Read the model definition and answer for the solid it produces. Units are mm, in the model's axes. A direction names the side the tool comes from. Round coordinates to 2 decimals unless told otherwise and drop trailing zeros. Write each loop counter-clockwise with the first axis right and the second up, starting at its lowest first coordinate (ties: lowest second). Pieces come first, ordered by that corner, then holes.
from build123d import *

# Parameters (mm, degrees)
F0_W     = 10
F0_H     = 10
F0_R     = 2.526739
F1_DEPTH = 1
F2_W     = 10
F2_H     = 1
F3_DEPTH = 9
F4_W     = 10
F4_H     = 1
F5_DEPTH = 9


with BuildPart() as f1:
    # F0 (on Top) → F1 (new body)
    with BuildSketch(Plane.XY):
        Rectangle(F0_W, F0_H)
        Circle(F0_R, mode=Mode.SUBTRACT)
    extrude(amount=F1_DEPTH)

    # F2 (on face) → F3 (join)
    with BuildSketch(Plane.XY.offset(1)):
        with Locations((0, 4.5)):
            Rectangle(F2_W, F2_H)
    extrude(amount=F3_DEPTH)

    # F4 (on face) → F5 (join)
    with BuildSketch(Plane.XZ.offset(-4)):
        with Locations((0, 9.5)):
            Rectangle(F4_W, F4_H)
    extrude(amount=F5_DEPTH)


solid = f1.part
Q1. Section D-D (x = -4) is taken. Determine the outline of the cut face in (y, z).
Verdict:
outline: (-5, 0) - (5, 0) - (5, 10) - (-5, 10) - (-5, 9) - (4, 9) - (4, 1) - (-5, 1) - close
Q2. Section B-B (x = 0) is taken. Determine the outline of the cut face in (y, z).
Verdict:
outline: (-5, 0) - (-2.53, 0) - (-2.53, 1) - (-5, 1) - close; (-5, 9) - (4, 9) - (4, 1) - (2.53, 1) - (2.53, 0) - (5, 0) - (5, 10) - (-5, 10) - close
Q3. A flat-ended cylindrical pin translates along its axis: pin 1 Ø4 at (x, z) = (-2, 4.5) entering from -Y. Find the tip coordinate at first contact, or state that the pin passes through.
Verdict:
pin 1: stops at y = 4
Q4. Section C-C (y = 2.75) is taken. Determine the outline of the cut face in (x, z).
Verdict:
outline: (-5, 0) - (5, 0) - (5, 1) - (-5, 1) - close; (-5, 9) - (5, 9) - (5, 10) - (-5, 10) - close
Q5. Which of the six approach directions +Z, -Z, +X, -X, +Y, -Y give full straight-line access (tool end or side, diameter ignored) to faces 5 (the flat face through (-0.1, -5, 0.5)), 6 (the flat face through (0, 0, 9))?
Verdict:
face 5: +Z, -Z, +X, -X, -Y
face 6: +X, -X, -Y
Q6. Straight lines are drawn through the part: probe 1 along Z at (x, y) = (4.25, 1.5); probe 2 along Y at (x, z) = (-2.75, 7.5); probe 3 along X at (y, z) = (2, 0.5). For each, find the intervals that lie inside material, in ascending order.
Verdict:
probe 1: z = 0 to 1, 9 to 10
probe 2: y = 4 to 5
probe 3: x = -5 to -1.54, 1.54 to 5
Q7. Determine the mould class of faces 1 (the flat face through (5, 4.5, 5.3)), 2 (the flat face through (-5, 4.5, 5.3)), 3 (the flat face through (0, 0, 10)), 4 (the cylindrical face through (-0.548, -2.467, 0.493)) for opening direction X: pulls with the +X half, pulls with the -X half, needs draft (parallel to the pull), parting line crosses it, or undercut.
Verdict:
face 1: pulls with the +X half
face 2: pulls with the -X half
face 3: needs draft
face 4: undercut
Q8. Section A-A (y = 0) is taken. Determine the outline of the cut face in (x, z), then the cut area to 3 significant figures.
Verdict:
outline: (-5, 0) - (-2.53, 0) - (-2.53, 1) - (-5, 1) - close; (-5, 9) - (5, 9) - (5, 10) - (-5, 10) - close; (2.53, 0) - (5, 0) - (5, 1) - (2.53, 1) - close
area: 14.9 mm2
